```python
from build123d import *

# Parameters (mm, degrees)
BOSS_EXTRUDE1_DEPTH = 3
SKETCH2_W           = 3
SKETCH2_H           = 15
CUT_EXTRUDE1_DEPTH  = 3
SKETCH3_R           = 7.5
CUT_EXTRUDE2_DEPTH  = 3


with BuildPart() as part:
    # Sketch1 → Boss-Extrude1 (new body)
    with BuildSketch(Plane.XY):
        with BuildLine():
            Line((10.455245645, 29.11454936), (110.455245645, 29.11454936))
            ThreePointArc((110.455245645, 29.11454936), (125.455245645, 14.11454936), (110.455245645, -0.88545064))
            Line((110.455245645, -0.88545064), (10.455245645, -0.88545064))
            ThreePointArc((10.455245645, -0.88545064), (-4.544754355, 14.11454936), (10.455245645, 29.11454936))
        make_face()
    extrude(amount=BOSS_EXTRUDE1_DEPTH)

    # Sketch2 → Cut-Extrude1 (cut)
    with BuildSketch(Plane.XY.offset(3)):
        with Locations((26.955245645, 6.61454936)):
            Rectangle(SKETCH2_W, SKETCH2_H)
        with Locations((93.955245645, 6.61454936)):
            Rectangle(SKETCH2_W, SKETCH2_H)
    extrude(amount=-CUT_EXTRUDE1_DEPTH, mode=Mode.SUBTRACT)

    # Sketch3 → Cut-Extrude2 (cut)
    with BuildSketch(Plane.XY.offset(3)):
        with Locations((10.455245645, 14.11454936)):
            Circle(SKETCH3_R)
        with Locations((110.455245645, 14.11454936)):
            Circle(SKETCH3_R)
    extrude(amount=-CUT_EXTRUDE2_DEPTH, mode=Mode.SUBTRACT)


solid = part.part
```
Geometry: final body of the model. Coordinates: model frame, mm. A direction names the side the tool comes from. Give positions to 0.01 mm unless a question says otherwise; leave off trailing zeros. Loops run counter-clockwise (first coordinate to the right, second up) from the corner with the lowest first, then second, coordinate; pieces in that order, holes last. Notation, with made-up numbers: (43.5, 65.25) -> (49.5, 65.25) arc R13 ccw to (49.5, 70.25) -> close; hole circle Ø8 at (-28, 3.5). An arc over 180 degrees is marked (long way). Return JSON: item names as keys, results as strings.
Item 1: Pin query (flat end, axial travel): P1, Ø0.9, axis at y = 10, z = 2, coming from the -X side; P2, Ø0.9, axis at x = 27.5, z = 2, coming from the -Y side; P3, Ø0.9, axis at y = 3.5, z = 1, coming from the +X side. Return the tip coordinate at first contact, or that it passes through.
Filled in:
{"P1": "x = -4.09", "P2": "y = 14.11", "P3": "x = 121.49"}
Item 2: Section D-D, the plane x = 27. Output: boundary loops of the cut face in (y, z), plus the area to 3 significant figures.
Filled in:
{"outline": "(14.11, 0) -> (29.11, 0) -> (29.11, 3) -> (14.11, 3) -> close", "area": "45.0 mm^2"}
Item 3: Section B-B, the plane y = 8.25. Output: boundary loops of the cut face in (x, z).
Filled in:
{"outline": "(-3.35, 0) -> (5.78, 0) -> (5.78, 3) -> (-3.35, 3) -> close; (15.13, 0) -> (25.46, 0) -> (25.46, 3) -> (15.13, 3) -> close; (28.46, 0) -> (92.46, 0) -> (92.46, 3) -> (28.46, 3) -> close; (95.46, 0) -> (105.78, 0) -> (105.78, 3) -> (95.46, 3) -> close; (115.13, 0) -> (124.26, 0) -> (124.26, 3) -> (115.13, 3) -> close"}
Item 4: Access query for faces 4 (the flat face through (103, -0.885, 1)), 5 (the flat face through (92.455, 7, 2)). Directions: +Z, -Z, +X, -X, +Y, -Y. A direction counts if a zero-diameter tool reaches every point of the face in a straight line with its end or side. Return the directions, or none.
Filled in:
{"face 4": "+Z, -Z, +X, -X, -Y", "face 5": "+Z, -Z, -Y"}
Item 5: Line query: line 1 (X direction, y = 16.25, z = 2.6); line 2 (X direction, y = 7.5, z = 0.9); line 3 (X direction, y = 17.5, z = 2.8). Output: solid intervals per line, ascending.
Filled in:
{"line 1": "-4.39 to 3.27, 17.64 to 103.27, 117.64 to 125.3", "line 2": "-3.01 to 6.92, 13.99 to 25.46, 28.46 to 92.46, 95.46 to 106.92, 113.99 to 123.92", "line 3": "-4.16 to 3.76, 17.15 to 103.76, 117.15 to 125.07"}
Item 6: Section A-A, the plane z = 0.7. Output: boundary loops of the cut face in (x, y).
Filled in:
{"outline": "(10.46, -0.89) -> (25.46, -0.89) -> (25.46, 14.11) -> (28.46, 14.11) -> (28.46, -0.89) -> (92.46, -0.89) -> (92.46, 14.11) -> (95.46, 14.11) -> (95.46, -0.89) -> (110.46, -0.89) arc R15 ccw to (110.46, 29.11) -> (10.46, 29.11) arc R15 ccw to start; hole circle Ø15 at (10.46, 14.11); hole circle Ø15 at (110.46, 14.11)"}
Item 7: Mould query, pull axis Y, two halves, no side actions, for faces 1 (the flat face through (28.455, 7, 2)), 2 (the flat face through (27, 14.115, 2)), 3 (the cylindrical face through (102.962, 14.444, 1.521)). Classes: released by +Y, released by -Y, zero draft, split by the parting line, or undercut.
Filled in:
{"face 1": "zero draft", "face 2": "released by -Y", "face 3": "undercut"}
Item 8: Section C-C, the plane x = 7. Output: boundary loops of the cut face in (y, z).
Filled in:
{"outline": "(-0.48, 0) -> (7.46, 0) -> (7.46, 3) -> (-0.48, 3) -> close; (20.77, 0) -> (28.71, 0) -> (28.71, 3) -> (20.77, 3) -> close"}
